from build123d import *

# Parameters (mm, degrees)
BOSS_EXTRU_1_DEPTH         = 3
ENL_V_MAT_EXTRU_1_DEPTH    = 1
ESQUISSE3_W                = 1
ESQUISSE3_H                = 46.165382348
BOSS_EXTRU_2_DEPTH         = 1
R_P_TITION_LIN_AIRE1_COUNT = 10
R_P_TITION_LIN_AIRE1_PITCH = 10
ESQUISSE4_W                = 115.142225127
ESQUISSE4_H                = 1
BOSS_EXTRU_3_DEPTH         = 1
R_P_TITION_LIN_AIRE2_COUNT = 4
R_P_TITION_LIN_AIRE2_PITCH = 9
ESQUISSE6_W                = 145.186811134
ESQUISSE6_H                = 82.250288406
ENL_V_MAT_EXTRU_2_DEPTH    = 4


with BuildPart() as part:
    # Esquisse1 → Boss.-Extru.1 (new body)
    with BuildSketch(Plane.XY):
        Polygon((-47.221929914, 24.410148906), (-29.387388435, -24.589851094), (53.691225904, -24.589851094), (62.331247959, 24.410148906), align=None)
        Polygon((-27.986973358, -22.589851094), (52.013026642, -22.589851094), (59.947740773, 22.410148906), (-44.3656339, 22.410148906), align=None, mode=Mode.SUBTRACT)
    extrude(amount=BOSS_EXTRU_1_DEPTH)

    # Esquisse2 → Enlèv. mat.-Extru.1 (cut)
    with BuildSketch(Plane.XY.offset(3)):
        Polygon((61.139494366, 23.410148906), (-45.793781907, 23.410148906), (-28.687180897, -23.589851094), (52.852126273, -23.589851094), align=None)
        Polygon((59.947740773, 22.410148906), (-44.3656339, 22.410148906), (-27.986973358, -22.589851094), (52.013026642, -22.589851094), align=None, mode=Mode.SUBTRACT)
    extrude(amount=-ENL_V_MAT_EXTRU_1_DEPTH, mode=Mode.SUBTRACT)

    # Esquisse3 → Boss.-Extru.2 (add)
    with BuildSketch(Plane.XY):
        with Locations((-37.740481402, -0.672542268)):
            Rectangle(ESQUISSE3_W, ESQUISSE3_H)
    boss_extru_2 = extrude(amount=BOSS_EXTRU_2_DEPTH)

    # Répétition linéaire1: Boss.-Extru.2 ×10
    with Locations(*[(i * R_P_TITION_LIN_AIRE1_PITCH, 0, 0) for i in range(1, R_P_TITION_LIN_AIRE1_COUNT)]):
        add(boss_extru_2)

    # Esquisse4 → Boss.-Extru.3 (add)
    with BuildSketch(Plane.XY):
        with Locations((11.695067266, 12.910148906)):
            Rectangle(ESQUISSE4_W, ESQUISSE4_H)
    boss_extru_3 = extrude(amount=BOSS_EXTRU_3_DEPTH)

    # Répétition linéaire2: Boss.-Extru.3 ×4
    with Locations(*[(0, -i * R_P_TITION_LIN_AIRE2_PITCH, 0) for i in range(1, R_P_TITION_LIN_AIRE2_COUNT)]):
        add(boss_extru_3)

    # Esquisse6 → Enlèv. mat.-Extru.2 (cut, through all)
    with BuildSketch(Plane.XY.offset(3)):
        with Locations((8.362981272, 0)):
            Rectangle(ESQUISSE6_W, ESQUISSE6_H)
        Polygon((62.331247959, 24.410148906), (-47.221929914, 24.410148906), (-29.387388435, -24.589851094), (53.691225904, -24.589851094), align=None, mode=Mode.SUBTRACT)
    extrude(amount=-ENL_V_MAT_EXTRU_2_DEPTH, mode=Mode.SUBTRACT)


solid = part.part
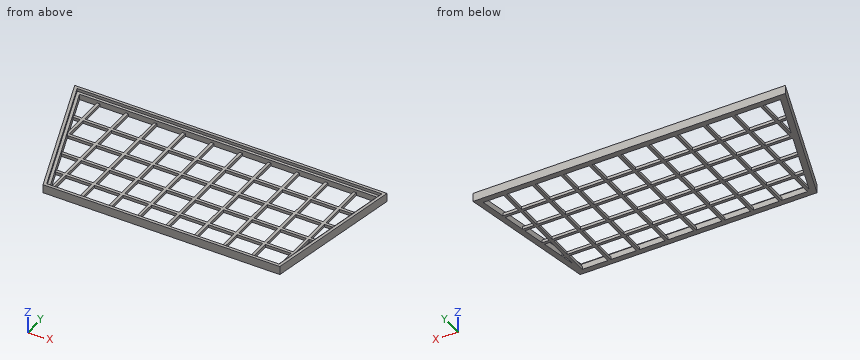
Read the model definition and answer for the solid it produces. Units are mm, in the model's axes. Give positions to 0.01 mm unless a question says otherwise; leave off trailing zeros. Write each loop counter-clockwise with the first axis right and the second up, starting at its lowest first coordinate (ties: lowest second). Pieces come first, ordered by that corner, then holes. Notation, with made-up numbers: (-23.5, -8.5) - (-1.5, -8.5) arc R12 ccw to (-1.5, 3.5) - close; hole circle Ø9 at (-12, -33). An arc over 180 degrees is marked (long way). Answer in a Markdown table with one row per item. Add a question column.
Item 1: Section B-B, the plane y = 0.5 is taken. Count the separate pieces of the cut face and the enclosed holes in it, and give its area (3 significant figures).
Item 2: Section A-A, the plane x = 24 is taken. Write down the section's boundary in (y, z), and give its area (3 significant figures).
Item 3: Find the intervals of material crossed by L1, parallel to Y at x = 44, z = 0.2; L2, parallel to Y at x = -17, z = 1.8; L3, parallel to Y at x = 48, z = 2.3, in increasing order.
Item 4: Flat-ended cylindrical pins translate along their axes: P1, Ø0.8, axis at y = -19.5, z = 0.5, coming from the +X side; P2, Ø0.8, axis at y = 20, z = 0.5, coming from the +X side; P3, Ø4, axis at x = -23.5, y = -11, coming from the +Z side; P4, Ø0.8, axis at y = -9.5, z = 0.5, coming from the +X side. Find the tip coordinate at first contact, or state that the pin passes through.
Recorded:
| question | item | result |
|---|---|---|
| 1 | separate pieces | 11 |
| 1 | enclosed holes | 0 |
| 1 | area | 19.4 mm2 |
| 2 | outline | (-24.59, 0) - (-22.59, 0) - (-22.59, 2) - (-23.59, 2) - (-23.59, 3) - (-24.59, 3) - close; (-14.59, 0) - (-13.59, 0) - (-13.59, 1) - (-14.59, 1) - close; (-5.59, 0) - (-4.59, 0) - (-4.59, 1) - (-5.59, 1) - close; (3.41, 0) - (4.41, 0) - (4.41, 1) - (3.41, 1) - close; (12.41, 0) - (13.41, 0) - (13.41, 1) - (12.41, 1) - close; (22.41, 0) - (24.41, 0) - (24.41, 3) - (23.41, 3) - (23.41, 2) - (22.41, 2) - close |
| 2 | area | 14.0 mm2 |
| 3 | L1 | y = -24.59 to -22.59, -14.59 to -13.59, -5.59 to -4.59, 3.41 to 4.41, 12.41 to 13.41, 22.41 to 24.41 |
| 3 | L2 | y = -24.59 to -22.59, 22.41 to 24.41 |
| 3 | L3 | y = -24.59 to -23.59, 23.41 to 24.41 |
| 4 | P1 | stops at x = 54.66 |
| 4 | P2 | stops at x = 61.62 |
| 4 | P3 | passes through |
| 4 | P4 | stops at x = 56.42 |
